Design review of the part built by this model. Coordinates are the model's own, in mm. A direction names the side the tool comes from. Round coordinates to 2 decimals unless told otherwise and drop trailing zeros. Order: outer loops, then holes, each group sorted by start corner. A loop starts at its lowest first (then second) coordinate and runs counter-clockwise, first axis right, second up.
from build123d import *

# Parameters (mm, degrees)
CUT_EXTRUDE_1_DEPTH = 2.5
FILLET_1_R          = 0.3
CHAMFER_1_SIZE      = 1.6


with BuildPart() as part:
    # Эскиз1 → Повернуть1 (revolve)
    with BuildSketch(Plane.XY):
        Polygon((0, 0), (0, 6.5), (8, 6.5), (8, 4), (38, 4), (38, 0), align=None)
    revolve(axis=Axis((38, 0, 0), (-1, 0, 0)))

    # Эскиз2 → Вырез-Вытянуть1 (cut)
    with BuildSketch(Plane.ZY):
        Polygon((-1.732050808, 3), (-3.464101615, 0), (-1.732050808, -3), (1.732050808, -3), (3.464101615, 0), (1.732050808, 3), align=None)
    extrude(amount=-CUT_EXTRUDE_1_DEPTH, mode=Mode.SUBTRACT)

    # Скругление1
    fillet_1_edges = [part.edges().sort_by_distance(p)[0] for p in [
        (8, -4, 0),
        (0, -6.5, 0),
    ]]
    fillet(fillet_1_edges, radius=FILLET_1_R)

    # Фаска1
    chamfer_1_edges = [part.edges().sort_by_distance(p)[0] for p in [
        (38, -4, 0),
    ]]
    chamfer(chamfer_1_edges, length=CHAMFER_1_SIZE)


solid = part.part
1) Take a section at A-A on z = 0. Give the boundary of the cut face in (x, y).
Results:
outline: (0, -6.2) arc R0.3 ccw to (0.3, -6.5) - (8, -6.5) - (8, -4.3) arc R0.3 cw to (8.3, -4) - (36.4, -4) - (38, -2.4) - (38, 2.4) - (36.4, 4) - (8.3, 4) arc R0.3 cw to (8, 4.3) - (8, 6.5) - (0.3, 6.5) arc R0.3 ccw to (0, 6.2) - (0, 3) - (2.5, 3) - (2.5, -3) - (0, -3) - close
2) Take a section at B-B on x = 7. Give the boundary of the cut face in (y, z).
Results:
outline: circle Ø13 at (0, 0)
3) For faces 1 (the face through (4.204, -5.158, 3.955)), 2 (the face through (8, 1.353, 4.242)), 3 (the face through (1, 3, 0)), list the 3-axis set-ups (+Z, -Z, +X, -X, +Y, -Y) from which the entire face can be reached by the end or side of a thin tool; tool diameter is ignored.
Results:
face 1: +X, -X
face 2: +X
face 3: -X
4) Take a section at C-C on x = 31. Give the boundary of the cut face in (y, z).
Results:
outline: circle Ø8 at (0, 0)
5) To check wall thickness, follow line 1 along X through (y, z) = (-3.5, -4.5); line 2 along Y through (x, z) = (18.5, 0); line 3 along Y through (x, z) = (30, -1.5). State the ranges of each line that lie inside material, in increasing order.
Results:
line 1: x = 0 to 8
line 2: y = -4 to 4
line 3: y = -3.71 to 3.71
6) Clearance check with flat-ended pins moving along their axes: P1, Ø2, axis at x = 17.5, y = -3, coming from the +Z side; P2, Ø3, axis at x = 1.5, z = -0.5, coming from the +Y side; P3, Ø3, axis at y = -0.5, z = 1, coming from the -X side; P4, Ø5, axis at x = 11.5, z = -4, coming from the -Y side. State where each tip first meets the part, or that it passes through.
Results:
P1: stops at z = 3.46
P2: stops at y = 6.5
P3: stops at x = 2.5
P4: stops at y = -3.71
7) The part is to be moulded in two halves that separate along Z. For faces 4 (the face through (22.547, -0.867, 3.905)), 5 (the face through (2.5, 0, 0)), 6 (the face through (0, 1.5, -2.8)), say which applies: released by +Z, released by -Z, zero draft, split by the parting line, or undercut.
Results:
face 4: split by the parting line
face 5: undercut
face 6: zero draft
